Part model, mm, in its own coordinate system. Face numbers are marked on the shaded views. A direction names the side the tool comes from. Coordinates: 2 decimals unless noted, no trailing zeros. Loops run counter-clockwise (first coordinate to the right, second up) from the corner with the lowest first, then second, coordinate; pieces in that order, holes last. Notation, with made-up numbers: (-27, -3.75) - (3, -3.75) arc R22 cw to (3, 30.25) - close; hole circle Ø1 at (-37.5, 84). An arc over 180 degrees is marked (long way). Use a Markdown table: item, result. Add a question column.
1) Drop flat-ended pins along their axis: P1, Ø3, axis at x = -411, z = -102, coming from the +Y side; P2, Ø5, axis at x = 221.5, y = 73, coming from the -Z side; P3, Ø5, axis at x = 122.5, z = -68.5, coming from the -Y side. Give the stop position or say it passes through.
2) Band-saw the part on C-C (z = -126.5). Give the cut face in (x, y), plus the area to 3 significant figures.
3) Probe probe 1 along Z at (x, y) = (-31, 681); probe 2 along Y at (x, z) = (107, -41.5); probe 3 along Y at (x, z) = (15.5, -76). List the from-to ranges inside material, lowest first. Write a range as [from, to].
4) Band-saw the part on A-A (x = 329). Give the cut face in (y, z), plus the area to 3 significant figures.
5) Tool access for the marked faces 1 and 2: list every direction of +Z, -Z, +X, -X, +Y, -Y with a clear straight run to the whole face (end or side of a thin tool).
6) Band-saw the part on B-B (y = 56.5). Give the cut face in (x, z).
Autodesk Inventor part; units mm, degrees
ref_plane "YZ Plane" through (0, 0, 0) normal (1, 0, 0) x (0, 1, 0)
ref_plane "XZ Plane" through (0, 0, 0) normal (0, 1, 0) x (-1, 0, 0)
ref_plane "XY Plane" through (0, 0, 0) normal (0, 0, 1) x (1, 0, 0)
sketch "Sketch1" plane through (0, 0, 0) normal (0, 0, 1) x (1, 0, 0)
  line L0 (-739.5, -950) -> (739.5, -950)
  line L1 (739.5, -950) -> (739.5, 950)
  line L2 (739.5, 950) -> (-739.5, 950)
  line L3 (-739.5, 950) -> (-739.5, -950)
  line L4 (-739.5, -950) -> (739.5, 950) construction
  line L5 (739.5, -950) -> (-739.5, 950) construction
  point P0 (0, 0)
  dimension "d0" = 1479
  dimension "d1" = 1900
extrude "Plate1" add sketch "Sketch1" along normal blind 3
sketch "Sketch3" plane through (-739.5, -947.8787, 0.8787) normal (0, -0.7071068, 0.7071068) x (1, 0, 0)
  line L0 (1479, 0) -> (0, 0)
  line L1 (0, 0) -> (0, -212)
  line L2 (0, -212) -> (1479, -212)
  line L3 (1479, -212) -> (1479, 0)
edge flange "Flange2" height 212 angle 45 thickness 3 bend radius 5 thickness toward (0, -0.7071068, 0.7071068) relief round relief width 3 relief depth 1.5 edges at (0, -950, 0) wall of the first edge with corners at (739.5, -947.8787, 0.8787) (-739.5, -947.8787, 0.8787) (-739.5, -1097.7853, -149.028) (739.5, -1097.7853, -149.028)
bend "Bend2"
corner "Corner2"
sketch "Sketch4" plane through (739.5, -1097.7853, -149.028) normal (0, 0.7071068, -0.7071068) x (-1, 0, 0)
  line L0 (1454, 36.661) -> (1454, 25) construction
  line L1 (1454, 25) -> (1254, 25) construction
  line L2 (1254, 25) -> (1254, 36.661) construction
  line L3 (1254, 36.661) -> (1454, 36.661) construction
  line L4 (0, 0) -> (1479, 0)
  line L5 (1479, 208.6863) -> (1479, 0)
  point P0 (739.5, 881.6301)
  point P1 (1454, 30.8305)
  dimension "d23" = 200
  dimension "d24" = 11.661
  dimension "d25" = 25
  dimension "d26" = 25
mark "Mark1"
equation "\"d2\" = Thickness"
equation "\"d13\" = BendReliefWidth"
equation "\"d14\" = BendReliefDepth"
equation "\"d15\" = MinimumRemnant"
equation "\"d16\" = TransitionRadius"
equation "\"d19\" = BendRadius"
equation "\"d20\" = CornerReliefSize"
equation "\"d21\" = GapSize"
equation "\"d22\" = JacobiRadiusSize"
equation "\"BendReliefWidth\" = Thickness"
equation "\"BendReliefDepth\" = 0.5 * Thickness"
equation "\"CornerReliefSize\" = 4 * Thickness"
equation "\"MinimumRemnant\" = 2 * Thickness"
equation "\"TransitionRadius\" = BendRadius"
equation "\"JacobiRadiusSize\" = BendRadius"
equation "\"GapSize\" = Thickness"
properties part number "BSH 012 floor" material "09g2s"
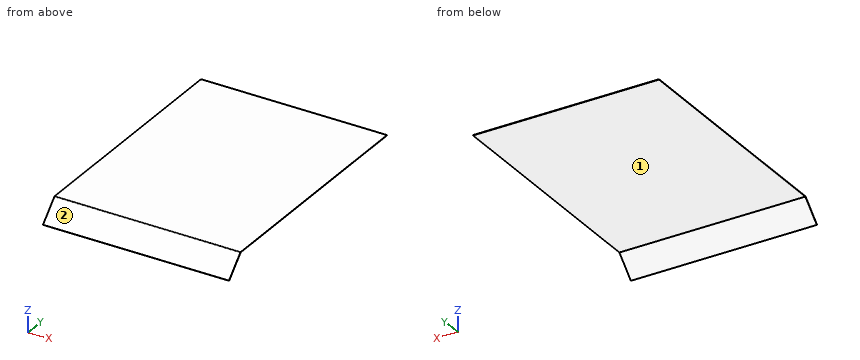
Answer block:
| question | item | result |
|---|---|---|
| 1 | P1 | y = -1049.26 |
| 1 | P2 | z = 0 |
| 1 | P3 | y = -1024 |
| 2 | outline | (-739.5, -1079.5) - (739.5, -1079.5) - (739.5, -1075.26) - (-739.5, -1075.26) - close |
| 2 | area | 6,270 mm2 |
| 3 | probe 1 | [0, 3] |
| 3 | probe 2 | [-994.5, -990.26] |
| 3 | probe 3 | [-1029, -1024.76] |
| 4 | outline | (-1099.91, -146.91) - (-1097.79, -149.03) - (-950.22, -1.46) arc R5 cw to (-946.69, 0) - (950, 0) - (950, 3) - (-946.69, 3) arc R8 ccw to (-952.34, 0.66) - close |
| 4 | area | 6,330 mm2 |
| 5 | face 1 | -Z, +X, -X, +Y |
| 5 | face 2 | +Z, +X, -X, -Y |
| 6 | outline | (-739.5, 0) - (739.5, 0) - (739.5, 3) - (-739.5, 3) - close |
